```python
from build123d import *

# Parameters (mm, degrees)
F0_W     = 31.75
F0_H     = 31.75
F1_DEPTH = 50.8
F2_W     = 19.05
F2_H     = 19.05
F3_DEPTH = 19.05
F4_W     = 15.875
F4_H     = 19.05
F5_DEPTH = 19.05
F7_DEPTH = 25.4
F9_DEPTH = 12.7


with BuildPart() as f1:
    # F0 (on Right) → F1 (new body)
    with BuildSketch(Plane.YZ):
        with Locations((15.875, 15.875)):
            Rectangle(F0_W, F0_H)
    extrude(amount=F1_DEPTH)

    # F2 (on face) → F3 (cut)
    with BuildSketch(Plane.XZ):
        with Locations((41.275, 22.225)):
            Rectangle(F2_W, F2_H)
    extrude(amount=-F3_DEPTH, mode=Mode.SUBTRACT)

    # F4 (on face) → F5 (cut)
    with BuildSketch(Plane.XZ):
        with Locations((7.9375, 22.225)):
            Rectangle(F4_W, F4_H)
    extrude(amount=-F5_DEPTH, mode=Mode.SUBTRACT)

    # F6 (on face) → F7 (cut)
    with BuildSketch(Plane.YZ.offset(31.75)):
        Polygon((0, 31.75), (0, 12.7), (19.05, 31.75), align=None)
    extrude(amount=-F7_DEPTH, mode=Mode.SUBTRACT)

    # F8 (on face) → F9 (cut)
    with BuildSketch(Plane.XZ.offset(-19.05)):
        Polygon((50.8, 12.7), (50.8, 31.75), (37.9892475903, 31.75), align=None)
    extrude(amount=-F9_DEPTH, mode=Mode.SUBTRACT)


solid = f1.part
```
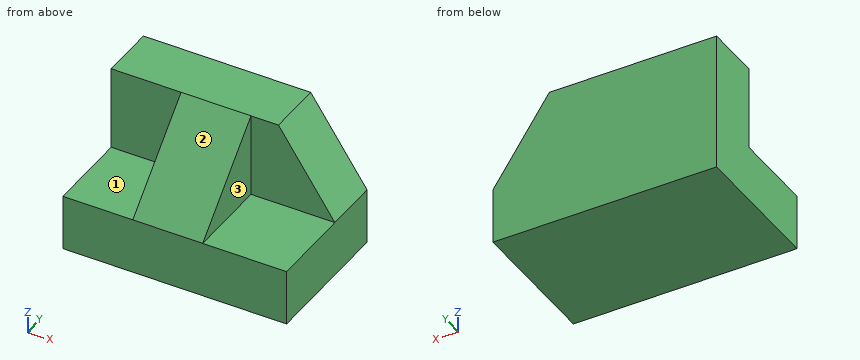
CAD build for the part. Positions are in the model's coordinates, mm. Face numbers are marked on the shaded views. A direction names the side the tool comes from. Coordinates: 2 decimals unless noted, no trailing zeros. Write each loop counter-clockwise with the first axis right and the second up, starting at its lowest first coordinate (ties: lowest second). Pieces come first, ordered by that corner, then holes. Notation, with made-up numbers: (66, -8) -> (104, -8) arc R33 cw to (104, 26) -> close; hole circle Ø10 at (78.5, -27.75). An arc over 180 degrees is marked (long way). Use CSV: the item, a comma, the result in double quotes. Start each with the question number.
Item 1: Tool access for the marked faces 1, 2 and 3: list every direction of +Z, -Z, +X, -X, +Y, -Y with a clear straight run to the whole face (end or side of a thin tool).
Item 2: Band-saw the part on B-B, the plane x = 22.5. Write the cut outline in (y, z).
Item 3: Band-saw the part on C-C, the plane z = 19.5. Write the cut outline in (x, y) (3 decimals), plus the area to 3 significant figures.
Item 4: Band-saw the part on D-D, the plane y = 29. Write the cut outline in (x, z), plus the area to 3 significant figures.
Item 5: Band-saw the part on A-A, the plane y = 16. Write the cut outline in (x, z) (3 decimals).
Item 6: Drop flat-ended pins along their axis: P1, Ø6, axis at x = 32, y = 6, coming from the -Z side; P2, Ø5, axis at y = 7.5, z = 24.5, coming from the +X side; P3, Ø6, axis at y = 10, z = 17.5, coming from the +X side; P4, Ø9.5, axis at x = 42, z = 21.5, coming from the -Y side. Give the stop position or say it passes through.
Item 7: Wall check: probe 1 along Y at (x, z) = (8.5, 18.5); probe 2 along X at (y, z) = (13.5, 17) (3 decimals); probe 3 along Z at (x, y) = (34, 19). Give the ranges that are in metal, low to high.
Response values:
1,face 1,"+Z, -X, -Y"
1,face 2,"+Z, +X, -X, -Y"
1,face 3,"+Z, +X, -Y"
2,outline,"(0, 0) -> (31.75, 0) -> (31.75, 31.75) -> (19.05, 31.75) -> (0, 12.7) -> close"
3,outline,"(0, 19.05) -> (15.875, 19.05) -> (15.875, 6.8) -> (31.75, 6.8) -> (31.75, 19.05) -> (46.227, 19.05) -> (46.227, 31.75) -> (0, 31.75) -> close"
3,area,"782 mm2"
4,outline,"(0, 0) -> (50.8, 0) -> (50.8, 12.7) -> (37.99, 31.75) -> (0, 31.75) -> close"
4,area,"1,490 mm2"
5,outline,"(0, 0) -> (50.8, 0) -> (50.8, 12.7) -> (31.75, 12.7) -> (31.75, 28.7) -> (15.875, 28.7) -> (15.875, 12.7) -> (0, 12.7) -> close"
6,P1,"stops at z = 0"
6,P2,"passes through"
6,P3,"stops at x = 31.75"
6,P4,"stops at y = 19.05"
7,probe 1,"y = 19.05 to 31.75"
7,probe 2,"x = 15.875 to 31.75"
7,probe 3,"z = 0 to 12.7"
